Part model, mm, in its own coordinate system. A direction names the side the tool comes from. Give positions to 0.01 mm unless a question says otherwise; leave off trailing zeros. Order: outer loops, then holes, each group sorted by start corner. A loop starts at its lowest first (then second) coordinate and runs counter-clockwise, first axis right, second up. Notation, with made-up numbers: (75.25, 21) - (94.25, 21) arc R19 cw to (94.25, 31) - close; hole circle Ø4 at (36.25, -36.5). An arc over 180 degrees is marked (long way). One line per item, written item: value.
Autodesk Inventor part; units mm, degrees
ref_plane "YZ Plane" through (0, 0, 0) normal (1, 0, 0) x (0, 1, 0)
ref_plane "XZ Plane" through (0, 0, 0) normal (0, 1, 0) x (-1, 0, 0)
ref_plane "XY Plane" through (0, 0, 0) normal (0, 0, 1) x (1, 0, 0)
sketch "Sketch1" plane through (0, 0, 0) normal (0, 0, 1) x (1, 0, 0)
  line L0 (0, 0) -> (19, 0)
  line L1 (19, 0) -> (19, 9)
  line L2 (19, 9) -> (0, 9)
  line L3 (0, 9) -> (0, 0)
  point P0 (9.5, 9)
  dimension "d0" = 19
  dimension "d1" = 9
extrude "Extrusion1" add sketch "Sketch1" along normal blind 3
sketch "Sketch2" plane through (0, 0, 3) normal (0, 0, 1) x (1, 0, 0)
  line L0 (19, 9) -> (0, 9)
  circle A0 centre (9.5, 7) radius 1
  point P0 (0, 0)
  point P1 (9.5, 9)
  dimension "d4" = 2
  dimension "d5" = 2
extrude "Extrusion2" add sketch "Sketch2" along normal blind 1.5
sketch "Sketch6" plane through (9.5, 7, 4.5) normal (0, 0, 1) x (1, 0, 0)
  circle A0 centre (0, 0) radius 1
  line L0 (2, -1) -> (-2, -1)
  line L1 (-2, -1) -> (-2, 1)
  line L2 (-2, 1) -> (2, 1)
  line L3 (2, 1) -> (2, -1)
  line L4 (2, -1) -> (-2, 1) construction
  line L5 (-2, -1) -> (2, 1) construction
  point P0 (-9.5, -7)
  dimension "d13" = 4
extrude "Extrusion5" add sketch "Sketch6" along normal blind 47
sketch "Sketch7" plane through (9.5, 7, 51.5) normal (0, 0, 1) x (1, 0, 0)
  circle A0 centre (0, 0) radius 1
  line L0 (-9.5, -7) -> (9.5, -7)
  line L1 (9.5, -7) -> (9.5, 2)
  line L2 (9.5, 2) -> (-9.5, 2)
  line L3 (-9.5, 2) -> (-9.5, -7)
  arc A1 (0, -1) -> (0, 1) centre (0, 0) ccw
  arc A2 (0, 1) -> (0, -1) centre (0, 0) ccw
extrude "Extrusion6" add sketch "Sketch7" along normal blind 4 contours A0 | L3 L2 L1 L0
sketch "Sketch8" plane through (9.5, 7, 55.5) normal (0, 0, 1) x (1, 0, 0)
  line L0 (-9.5, -7) -> (9.5, -7)
  line L1 (9.5, -7) -> (9.5, 2)
  line L2 (9.5, 2) -> (-9.5, 2)
  line L3 (-9.5, 2) -> (-9.5, -7)
  circle A0 centre (0, -3.5) radius 1.65
  dimension "d18" = 3.3
  dimension "d66" = 5.5
extrude "Extrusion7" cut sketch "Sketch8" against normal blind 4 contours A0
sketch "Sketch10" plane through (0, 0, 0) normal (-1, 0, 0) x (0, 0, 1)
  line L0 (0, 0) -> (3, 0)
  line L1 (3, 9) -> (3, 0)
  line L2 (3, 0) -> (2, 0)
  line L3 (2, 0) -> (2, 6)
  line L4 (2, 6) -> (3, 6)
  line L5 (3, 6) -> (3, 0)
  line L6 (3, 0) -> (2, 1)
  line L7 (3, 0) -> (4.4142, 0) construction
  line L8 (2, 1) -> (3, 2)
  line L9 (3, 0) -> (3, 9)
  line L10 (3, 2) -> (2, 3)
  line L11 (2, 3) -> (3, 4)
  line L12 (2, 5) -> (3, 4)
  line L13 (2, 5) -> (3, 6)
  dimension "d23" = 1
  dimension "d24" = 6
  dimension "d25" = 135
  dimension "d26" = 90
extrude "Extrusion8" cut sketch "Sketch10" against normal up to next contours L6 L8 L1 | L10 L11 L1 | L12 L13 L1
sketch "Sketch11" plane through (0, 0, 0) normal (0, -1, 0) x (1, 0, 0)
  line L0 (0, 3) -> (9.5, 3)
  line L1 (0, 3) -> (19, 3)
  line L2 (19, 3) -> (19, 2)
  line L3 (19, 2) -> (8.5, 2)
  line L4 (0, 2) -> (0, 3)
  line L5 (0, 3) -> (0, 2)
  line L6 (0, 3) -> (1.4142, 3) construction
  line L7 (19, 3) -> (0, 3)
  line L8 (9.5, 3) -> (8.5, 2)
  line L9 (9.5, 3) -> (10.9142, 3) construction
  line L10 (10.5, 2) -> (8.5, 2)
  line L11 (9.5, 3) -> (10.5, 2)
  line L12 (10.5, 2) -> (8.5, 2)
  line L13 (8.5, 2) -> (0, 2)
  line L14 (7.5, 3) -> (8.5, 2)
  line L15 (8.5, 2) -> (6.5, 2)
  line L16 (7.5, 3) -> (6.5, 2)
  line L17 (5.5, 3) -> (6.5, 2)
  line L18 (6.5, 2) -> (4.5, 2)
  line L19 (5.5, 3) -> (4.5, 2)
  line L20 (3.5, 3) -> (4.5, 2)
  line L21 (4.5, 2) -> (2.5, 2)
  line L22 (3.5, 3) -> (2.5, 2)
  line L23 (12.5, 2) -> (10.5, 2)
  line L24 (11.5, 3) -> (12.5, 2)
  line L25 (11.5, 3) -> (10.5, 2)
  line L26 (14.5, 2) -> (12.5, 2)
  line L27 (13.5, 3) -> (14.5, 2)
  line L28 (13.5, 3) -> (12.5, 2)
  line L29 (16.5, 2) -> (14.5, 2)
  line L30 (15.5, 3) -> (16.5, 2)
  line L31 (15.5, 3) -> (14.5, 2)
  point P0 (0, 0)
  dimension "d36" = 10
  dimension "d30" = 135
  dimension "d33" = 2
  dimension "d40" = 2
extrude "Extrusion9" cut sketch "Sketch11" against normal blind 6 contours L0 L22 L13 L4 | L0 L19 L20 | L0 L16 L17 | L0 L8 L14 | L1 L25 L11 | L1 L28 L24 | L1 L31 L27 | L1 L2 L3 L30
fillet "Fillet2" radius 1 4 edges at (19, 0, 1) (19, 9, 1.5) (0, 0, 1) (0, 9, 1.5)
fillet "Fillet3" radius 2 4 edges at (19, 0, 53.5) (19, 9, 53.5) (0, 0, 53.5) (0, 9, 53.5)
extrude "Extrusion10" add sketch "Sketch6" against normal up to surface (1.5 mm away) contours A0 L2 L3 L0 | A0 L0 L1 L2
sketch "Sketch12" plane through (9.5, 7, 51.5) normal (0, 0, -1) x (-1, 0, 0)
  circle A0 centre (0, 0) radius 1
  line L0 (-2, 1) -> (-2, -1)
  line L1 (-2, -1) -> (2, -1)
  line L2 (2, 1) -> (-2, 1)
  line L3 (2, -1) -> (2, 1)
  point P0 (9.5, -7)
extrude "Extrusion11" cut sketch "Sketch12" along normal blind 4 contours A0 L2 L3 L1 | A0 L1 L0 L2
chamfer "Chamfer3" distance 2 distance2 1 1 edges at (7.5, 7, 47.5) measured on face at (7.5, 7.3333, 32.6667)
chamfer "Chamfer4" distance 2 distance2 1 1 edges at (11.5, 7, 47.5) measured on face at (11.5, 6.6667, 32.6667)
properties part number "Clamp-part1-Base9x19mm-narrowTOP-maxSample40mm"
1) Slice it at B-B on z = 49.5. Write the cut outline in (x, y), then the cut area to 3 significant figures.
Answer:
outline: circle Ø2 at (9.5, 7)
area: 3.14 mm2
2) Slice it at A-A on y = 3.5. Count the separate pieces of the cut face and the enclosed holes in it, then the cut area to 3 significant figures.
Answer:
separate pieces: 3
enclosed holes: 0
area: 106 mm2
3) Which spindle directions (+Z, -Z, +X, -X, +Y, -Y) get a long thin tool onto all of the face, cutting with end or side? Do faces 1 (the face through (3.5, 3.4, 2.4)), 2 (the face through (6.8, 5.7, 2.3)), 3 (the face through (2.9, 4, 2.4)), 4 (the face through (16.2, 0.3, 2.3)), 5 (the face through (9.5, 3.4, 2.4)). Say none if no direction does.
Answer:
face 1: +X, -X
face 2: -Y
face 3: -X, -Y
face 4: +X, -Y
face 5: +Z, +X, -X
4) Slice it at C-C on z = 7. Write the cut outline in (x, y), then the cut area to 3 significant figures.
Answer:
outline: (7.5, 6) - (11.5, 6) - (11.5, 8) - (7.5, 8) - close
area: 8.00 mm2
5) Wall check: line 1 along Y through (x, z) = (9.5, 52.6); line 2 along Z through (x, y) = (10.25, 8.25); line 3 along Z through (x, y) = (10.5, 1). Give the ranges that are in metal, low to high. Write a range as [from, to].
Answer:
line 1: y = [0, 1.85], [5.15, 9]
line 2: z = [0, 3], [51.5, 55.5]
line 3: z = [0, 2], [51.5, 55.5]
6) Two-plate mould, pull along X, no slides. Class faces 6 (the face through (14.1, 4, 2.4)), 7 (the face through (18.715, 8.699, 1.521)), 8 (the face through (1, 3, 2)): pulls with the +X half, pulls with the -X half, needs draft (parallel to the pull), parting line crosses it, or undercut.
Answer:
face 6: undercut
face 7: pulls with the +X half
face 8: needs draft
7) Drop flat-ended pins along their axis: P1, Ø2, axis at y = 7.5, z = 23.5, coming from the +X side; P2, Ø0.8, axis at x = 1.5, z = 2.5, coming from the -Y side; P3, Ø3, axis at x = 7.5, z = 10, coming from the +Y side. Give the stop position or say it passes through.
Answer:
P1: stops at x = 11.5
P2: stops at y = 6
P3: stops at y = 8
